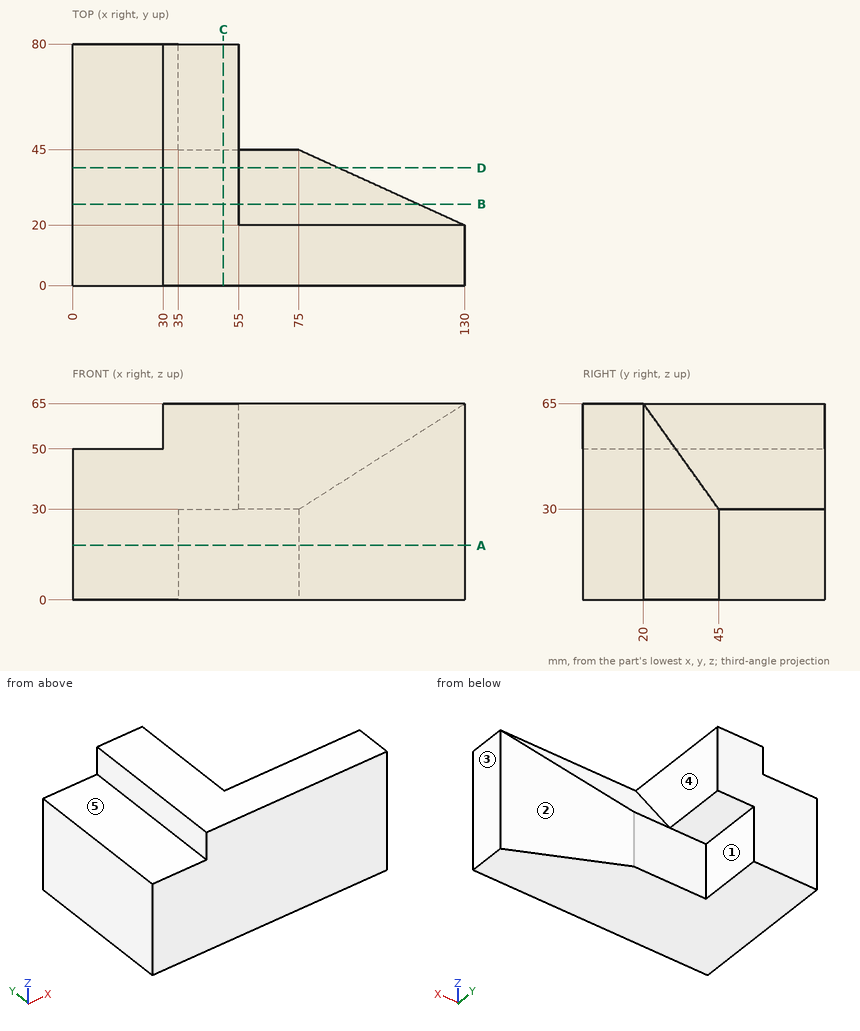
Verification items for this drawing (mm, ordinates from the low corner). A direction names the side the tool comes from. Coordinates: 2 decimals unless noted, no trailing zeros. Order: outer loops, then holes, each group sorted by start corner. A loop starts at its lowest first (then second) coordinate and runs counter-clockwise, first axis right, second up. Notation, with made-up numbers: M 87.5,28 L 132.5,28 A16 ccw 132.5,53 Z; hole C -36,51 d7. An arc over 180 degrees is marked long. Answer as a JSON object with one key per item and string values.
Q1. Tool access check on the marked faces 1, 2, 3, 4 and 5. Record the directions out of +Z, -Z, +X, -X, +Y, -Y that give a thin tool (end or side, any length) a straight path to the whole face; none if there is none.
Results are:
{"face 1": "-Z, +X, +Y", "face 2": "+Z, -Z, +X, +Y", "face 3": "+Z, -Z, +X, +Y, -Y", "face 4": "+Z, +X, +Y", "face 5": "+Z, -X, +Y, -Y"}
Q2. Scan lines: line 1 (Z direction, x = 10, y = 41); line 2 (X direction, y = 47.5, z = 12); line 3 (X direction, y = 44, z = 60.5). Record each from-to range of solid material in increasing order.
Results are:
{"line 1": "z = 0 to 50", "line 2": "x = 0 to 35", "line 3": "x = 30 to 55"}
Q3. Cross-section at C-C on x = 50. Record the cut outline in (y, z).
Results are:
{"outline": "M 0,0 L 45,0 L 45,30 L 80,30 L 80,65 L 0,65 Z"}
Q4. Cross-section at A-A on z = 18. Record the cut outline in (x, y).
Results are:
{"outline": "M 0,0 L 130,0 L 130,20 L 75,45 L 35,45 L 35,80 L 0,80 Z"}
Q5. Cross-section at D-D on y = 39. Record the cut outline in (x, z), and give its area (3 significant figures).
Results are:
{"outline": "M 0,0 L 88.2,0 L 88.2,38.4 L 55,38.4 L 55,65 L 30,65 L 30,50 L 0,50 Z", "area": "4,400 mm²"}
Q6. Depth check by flat-ended pin: pin 1 Ø9 at (y, z) = (63, 8.5) entering from +X; pin 2 Ø12 at (y, z) = (58, 59.5) entering from -X; pin 3 Ø6 at (x, z) = (109.5, 46) entering from +Y. Enter the tip coordinate at first touch or a pass-through.
Results are:
{"pin 1": "stops at x = 35", "pin 2": "stops at x = 30", "pin 3": "stops at y = 30.68"}
Q7. Cross-section at B-B on y = 27. Record the cut outline in (x, z).
Results are:
{"outline": "M 0,0 L 114.6,0 L 114.6,55.2 L 55,55.2 L 55,65 L 30,65 L 30,50 L 0,50 Z"}
